The listing builds one solid part. Answer for the finished solid, in the listing's coordinates (mm). Coordinates: 2 decimals unless noted, no trailing zeros.
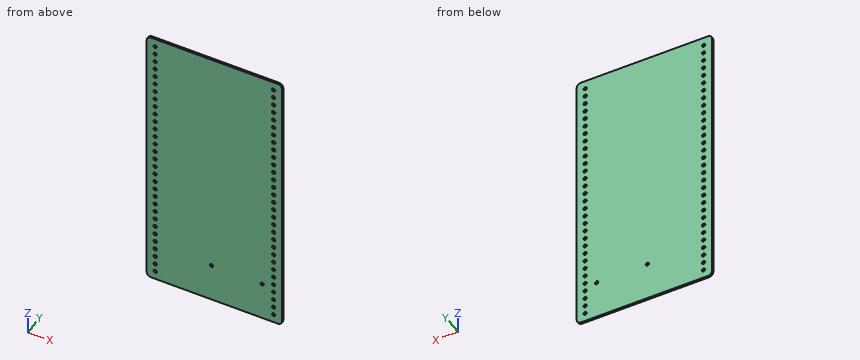
from build123d import *

# Parameters (mm, degrees)
BOSS_EXTRUDE1_DEPTH = 3.175
SKETCH3_R           = 2.5
CUT_EXTRUDE2_DEPTH  = 4.175
SKETCH7_R           = 2.5
CUT_EXTRUDE5_DEPTH  = 4.175


with BuildPart() as part:
    # Sketch1 → Boss-Extrude1 (new body)
    with BuildSketch(Plane(origin=(0, 0, 0), x_dir=(1, 0, 0), z_dir=(0, 1, 0))):
        with BuildLine():
            Line((-77.88977591, 288.008963585), (112.61022409, 288.008963585))
            ThreePointArc((112.61022409, 288.008963585), (117.10035215, 286.149091646), (118.96022409, 281.658963585))
            Line((118.96022409, 281.658963585), (118.96022409, -112.041036415))
            ThreePointArc((118.96022409, -112.041036415), (117.10035215, -116.531164475), (112.61022409, -118.391036415))
            Line((112.61022409, -118.391036415), (-77.88977591, -118.391036415))
            ThreePointArc((-77.88977591, -118.391036415), (-82.379903971, -116.531164475), (-84.23977591, -112.041036415))
            Line((-84.23977591, -112.041036415), (-84.23977591, 281.658963585))
            ThreePointArc((-84.23977591, 281.658963585), (-82.379903971, 286.149091646), (-77.88977591, 288.008963585))
        make_face()
    extrude(amount=BOSS_EXTRUDE1_DEPTH)

    # Sketch3 → Cut-Extrude2 (cut, through all)
    with BuildSketch(Plane(origin=(0, 3.175, 0), x_dir=(1, 0, 0), z_dir=(0, 1, 0))):
        with Locations((-71.53977591, 275.308963585)):
            Circle(SKETCH3_R)
        with Locations((106.26022409, 275.308963585)):
            Circle(SKETCH3_R)
        with Locations((-71.53977591, 262.608963585)):
            Circle(SKETCH3_R)
        with Locations((106.26022409, 262.608963585)):
            Circle(SKETCH3_R)
        with Locations((-71.53977591, 249.908963585)):
            Circle(SKETCH3_R)
        with Locations((106.26022409, 249.908963585)):
            Circle(SKETCH3_R)
        with Locations((-71.53977591, 237.208963585)):
            Circle(SKETCH3_R)
        with Locations((106.26022409, 237.208963585)):
            Circle(SKETCH3_R)
        with Locations((-71.53977591, 224.508963585)):
            Circle(SKETCH3_R)
        with Locations((106.26022409, 224.508963585)):
            Circle(SKETCH3_R)
        with Locations((-71.53977591, 211.808963585)):
            Circle(SKETCH3_R)
        with Locations((106.26022409, 211.808963585)):
            Circle(SKETCH3_R)
        with Locations((-71.53977591, 199.108963585)):
            Circle(SKETCH3_R)
        with Locations((106.26022409, 199.108963585)):
            Circle(SKETCH3_R)
        with Locations((-71.53977591, 186.408963585)):
            Circle(SKETCH3_R)
        with Locations((106.26022409, 186.408963585)):
            Circle(SKETCH3_R)
        with Locations((-71.53977591, 173.708963585)):
            Circle(SKETCH3_R)
        with Locations((106.26022409, 173.708963585)):
            Circle(SKETCH3_R)
        with Locations((-71.53977591, 161.008963585)):
            Circle(SKETCH3_R)
        with Locations((106.26022409, 161.008963585)):
            Circle(SKETCH3_R)
        with Locations((-71.53977591, 148.308963585)):
            Circle(SKETCH3_R)
        with Locations((106.26022409, 148.308963585)):
            Circle(SKETCH3_R)
        with Locations((-71.53977591, 135.608963585)):
            Circle(SKETCH3_R)
        with Locations((106.26022409, 135.608963585)):
            Circle(SKETCH3_R)
        with Locations((-71.53977591, 122.908963585)):
            Circle(SKETCH3_R)
        with Locations((106.26022409, 122.908963585)):
            Circle(SKETCH3_R)
        with Locations((-71.53977591, 110.208963585)):
            Circle(SKETCH3_R)
        with Locations((106.26022409, 110.208963585)):
            Circle(SKETCH3_R)
        with Locations((-71.53977591, 97.508963585)):
            Circle(SKETCH3_R)
        with Locations((106.26022409, 97.508963585)):
            Circle(SKETCH3_R)
        with Locations((-71.53977591, 84.808963585)):
            Circle(SKETCH3_R)
        with Locations((106.26022409, 84.808963585)):
            Circle(SKETCH3_R)
        with Locations((-71.53977591, 72.108963585)):
            Circle(SKETCH3_R)
        with Locations((106.26022409, 72.108963585)):
            Circle(SKETCH3_R)
        with Locations((-71.53977591, 59.408963585)):
            Circle(SKETCH3_R)
        with Locations((106.26022409, 59.408963585)):
            Circle(SKETCH3_R)
        with Locations((-71.53977591, 46.708963585)):
            Circle(SKETCH3_R)
        with Locations((106.26022409, 46.708963585)):
            Circle(SKETCH3_R)
        with Locations((-71.53977591, 34.008963585)):
            Circle(SKETCH3_R)
        with Locations((106.26022409, 34.008963585)):
            Circle(SKETCH3_R)
        with Locations((-71.53977591, 21.308963585)):
            Circle(SKETCH3_R)
        with Locations((106.26022409, 21.308963585)):
            Circle(SKETCH3_R)
        with Locations((-71.53977591, 8.608963585)):
            Circle(SKETCH3_R)
        with Locations((106.26022409, 8.608963585)):
            Circle(SKETCH3_R)
        with Locations((-71.53977591, -4.091036415)):
            Circle(SKETCH3_R)
        with Locations((106.26022409, -4.091036415)):
            Circle(SKETCH3_R)
        with Locations((-71.53977591, -16.791036415)):
            Circle(SKETCH3_R)
        with Locations((106.26022409, -16.791036415)):
            Circle(SKETCH3_R)
        with Locations((-71.53977591, -29.491036415)):
            Circle(SKETCH3_R)
        with Locations((106.26022409, -29.491036415)):
            Circle(SKETCH3_R)
        with Locations((-71.53977591, -42.191036415)):
            Circle(SKETCH3_R)
        with Locations((106.26022409, -42.191036415)):
            Circle(SKETCH3_R)
        with Locations((-71.53977591, -54.891036415)):
            Circle(SKETCH3_R)
        with Locations((106.26022409, -54.891036415)):
            Circle(SKETCH3_R)
        with Locations((-71.53977591, -67.591036415)):
            Circle(SKETCH3_R)
        with Locations((106.26022409, -67.591036415)):
            Circle(SKETCH3_R)
        with Locations((-71.53977591, -80.291036415)):
            Circle(SKETCH3_R)
        with Locations((106.26022409, -80.291036415)):
            Circle(SKETCH3_R)
        with Locations((-71.53977591, -92.991036415)):
            Circle(SKETCH3_R)
        with Locations((106.26022409, -92.991036415)):
            Circle(SKETCH3_R)
        with Locations((-71.53977591, -105.691036415)):
            Circle(SKETCH3_R)
        with Locations((106.26022409, -105.691036415)):
            Circle(SKETCH3_R)
    extrude(amount=-CUT_EXTRUDE2_DEPTH, mode=Mode.SUBTRACT)

    # Sketch7 → Cut-Extrude5 (cut, through all)
    with BuildSketch(Plane(origin=(0, 3.175, 0), x_dir=(1, 0, 0), z_dir=(0, 1, 0))):
        with Locations((89.075893655, 230.566598453)):
            Circle(SKETCH7_R)
        with Locations((12.875893655, 230.566598453)):
            Circle(SKETCH7_R)
    extrude(amount=-CUT_EXTRUDE5_DEPTH, mode=Mode.SUBTRACT)


solid = part.part
Q1. Given pin 1 (4 mm diameter, centred on x = -71.54, z = -122.91, fed in from -Y); pin 2 (8 mm diameter, centred on x = -71.54, z = -199.11, fed in from +Y) (3 decimals), each flat-ended and moving along its own axis, determine where each tip first touches the part or whether it passes through.
Answers below:
pin 1: passes through
pin 2: stops at y = 3.175
Q2. The part is cut by section A-A, the plane y = 0.75. State how many separate pieces and enclosed holes the cut face has, then the cut area to 3 significant figures.
Answers below:
separate pieces: 1
enclosed holes: 64
area: 81,300 mm2
Q3. Find the intervals of material crossed by probe 1 along X at (y, z) = (0.85, 18); probe 2 along X at (y, z) = (0.8, -33.5); probe 3 along Z at (x, y) = (13.5, 1.6), in increasing order.
Answers below:
probe 1: x = -84.24 to -73.73, -69.35 to 104.07, 108.45 to 118.96
probe 2: x = -84.24 to -73.99, -69.09 to 103.81, 108.71 to 118.96
probe 3: z = -288.01 to -232.99, -228.15 to 118.39
